For this review, use the dimensioned drawing (mm, ordinates from the lowest corner) and the shaded views. A direction names the side the tool comes from. Round coordinates to 2 decimals unless told otherwise and drop trailing zeros. Write each loop counter-clockwise with the first axis right and the second up, starting at its lowest first coordinate (ties: lowest second). Pieces come first, ordered by that corner, then holes.
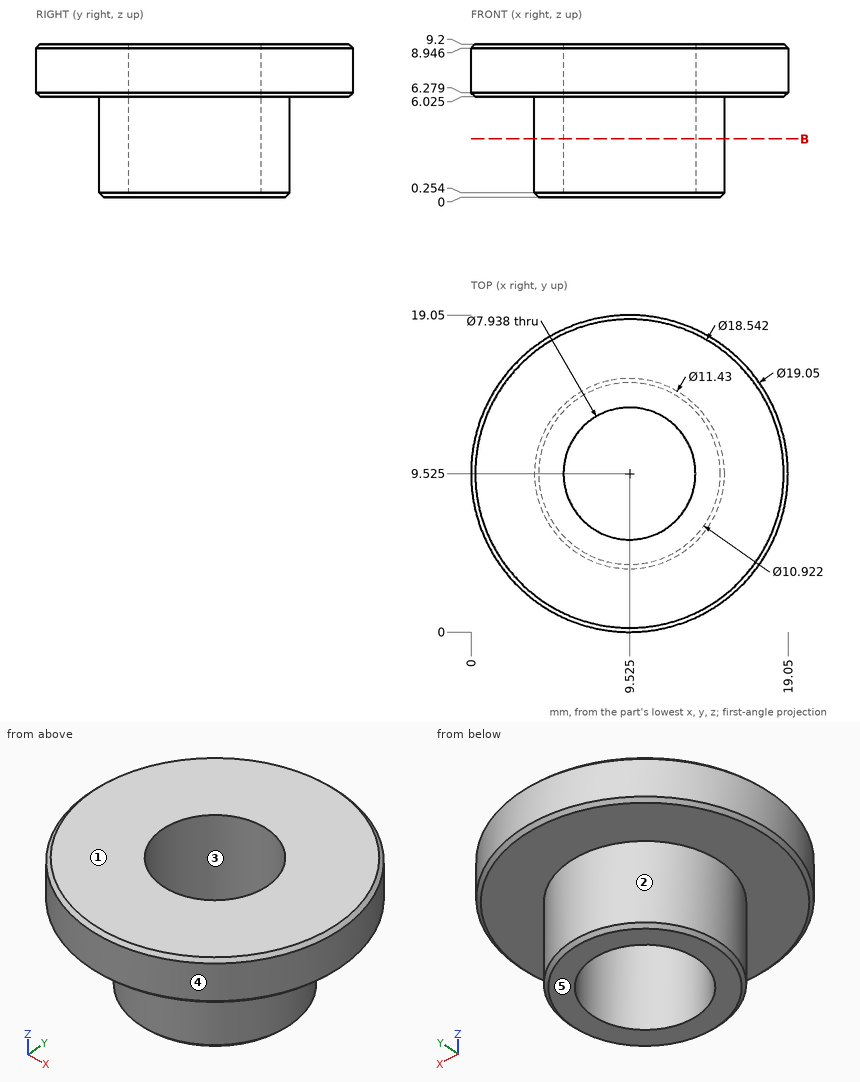
(1) Mouldability with a two-part tool opening along X and no side actions: class the marked faces 3, 4 and 5 as pulls with the +X half, pulls with the -X half, needs draft (parallel to the pull), parting line crosses it, or undercut.
Geometry check:
face 3: undercut
face 4: parting line crosses it
face 5: needs draft
(2) For pin 1 Ø5 at (y, z) = (15.5, 8) entering from +X; pin 2 Ø5 at (x, z) = (7, 5) entering from +Y, all flat-tipped, find the tip position at first contact; note any pin that passes through.
Geometry check:
pin 1: stops at x = 18.39
pin 2: stops at y = 19.04
(3) For line 1 along Z through (x, y) = (4.5, 14.25) (1 decimal); line 2 along X through (y, z) = (7.75, 7.5) (1 decimal); line 3 along X through (y, z) = (11.5, 3.75), list the stretches that pass through material, from the lowest coordinate up.
Geometry check:
line 1: z = 6 to 9.2
line 2: x = 0.2 to 6, 13.1 to 18.9
line 3: x = 4.16 to 6.08, 12.97 to 14.89
(4) For the marked faces 1 and 2, list the 3-axis set-ups (+Z, -Z, +X, -X, +Y, -Y) from which the entire face can be reached by the end or side of a thin tool; tool diameter is ignored.
Geometry check:
face 1: +Z, +X, -X, +Y, -Y
face 2: -Z
(5) We need section B-B, the plane z = 3.5. Give the boundary of the cut face in (x, y) (1 decimal).
Geometry check:
outline: circle Ø11.4 at (9.5, 9.5); hole circle Ø7.9 at (9.5, 9.5)
